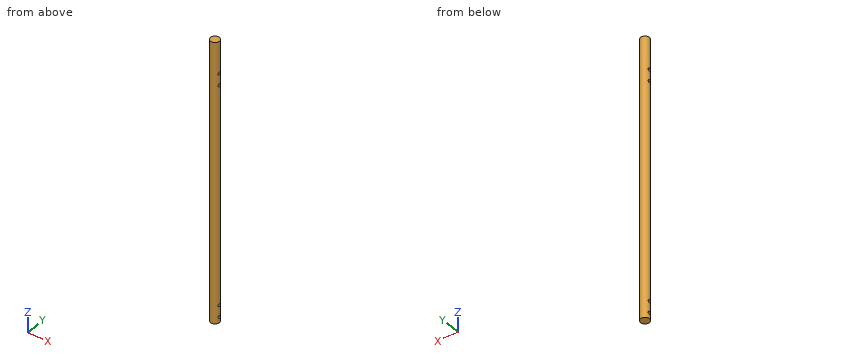
from build123d import *

# Parameters (mm, degrees)
SKETCH1_R                       = 9.525
BOSS_EXTRUDE1_DEPTH             = 609.6
F_1_4_0_25_DIAMETER_HOLE1_D     = 6.35
F_1_4_0_25_DIAMETER_HOLE1_DEPTH = 25.399
F_1_4_0_25_DIAMETER_HOLE1_TIP   = 1.907732465
F_1_4_0_25_DIAMETER_HOLE2_D     = 6.35
F_1_4_0_25_DIAMETER_HOLE2_DEPTH = 25.4
F_1_4_0_25_DIAMETER_HOLE2_TIP   = 1.907732465


with BuildPart() as part:
    # Sketch1 → Boss-Extrude1 (new body)
    with BuildSketch(Plane.XY):
        with Locations(Location((0, 0, 0), (0, 0, 180))):
            Circle(SKETCH1_R)
    extrude(amount=BOSS_EXTRUDE1_DEPTH)

    # 1/4 (0.25) Diameter Hole1
    with Locations(Plane(origin=(-12.7, 0, 514.35), x_dir=(0, 0, -1), z_dir=(-1, 0, 0))):
        with Locations((0, 0), (-25.4, 0)):
            Hole(F_1_4_0_25_DIAMETER_HOLE1_D / 2, depth=F_1_4_0_25_DIAMETER_HOLE1_DEPTH)
            with Locations((0, 0, -(F_1_4_0_25_DIAMETER_HOLE1_DEPTH + F_1_4_0_25_DIAMETER_HOLE1_TIP / 2))):  # 118° drill point
                Cone(0, F_1_4_0_25_DIAMETER_HOLE1_D / 2, F_1_4_0_25_DIAMETER_HOLE1_TIP, mode=Mode.SUBTRACT)

    # 1/4 (0.25) Diameter Hole2
    with Locations(Plane(origin=(-12.7, 0, 38.1), x_dir=(0, 0, -1), z_dir=(-1, 0, 0))):
        with Locations((0, 0), (25.4, 0)):
            Hole(F_1_4_0_25_DIAMETER_HOLE2_D / 2, depth=F_1_4_0_25_DIAMETER_HOLE2_DEPTH)
            with Locations((0, 0, -(F_1_4_0_25_DIAMETER_HOLE2_DEPTH + F_1_4_0_25_DIAMETER_HOLE2_TIP / 2))):  # 118° drill point
                Cone(0, F_1_4_0_25_DIAMETER_HOLE2_D / 2, F_1_4_0_25_DIAMETER_HOLE2_TIP, mode=Mode.SUBTRACT)


solid = part.part
Input: part model. Units: mm. Frame: model coordinates. Round coordinates to 2 decimals unless told otherwise and drop trailing zeros. Write each loop counter-clockwise with the first axis right and the second up, starting at its lowest first coordinate (ties: lowest second). Pieces come first, ordered by that corner, then holes.
1) Contact query for flat-ended pins moving along their axis: P1, Ø8, axis at y = -5, z = 194.5, coming from the -X side; P2, Ø1, axis at y = -4.5, z = 337.5, coming from the -X side; P3, Ø1.5, axis at y = -6.5, z = 63.5, coming from the -X side. Output: stop coordinate, or through.
2) Cut plane B-B (x = 1.75). Return the cut outline in (y, z) (3 decimals), then the cut area to 3 significant figures.
3) Cut plane C-C (z = 149.5). Return the cut outline in (x, y) (3 decimals), then the cut area to 3 significant figures.
4) Cut plane A-A (y = 0). Return the cut outline in (x, z) (3 decimals), then the cut area to 3 significant figures.
5) Ray query, L1, parallel to Y at x = -0.25, z = 514.35 (3 decimals); L2, parallel to Z at x = 2.5, y = 1.5; L3, parallel to X at y = -0.25, z = 519. Return the intervals inside material, ascending.
Geometry says:
1. P1: stops at x = -9.47
1. P2: stops at x = -8.64
1. P3: stops at x = -7.59
2. outline: (-9.363, 0) - (9.363, 0) - (9.363, 609.6) - (-9.363, 609.6) - close; hole circle Ø6.35 at (0, 12.7); hole circle Ø6.35 at (0, 38.1); hole circle Ø6.35 at (0, 514.35); hole circle Ø6.35 at (0, 539.75)
2. area: 11,300 mm2
3. outline: circle Ø19.05 at (0, 0)
3. area: 285 mm2
4. outline: (-9.525, 0) - (9.525, 0) - (9.525, 9.525) - (-9.525, 9.525) - close; (-9.525, 15.875) - (9.525, 15.875) - (9.525, 34.925) - (-9.525, 34.925) - close; (-9.525, 41.275) - (9.525, 41.275) - (9.525, 511.175) - (-9.525, 511.175) - close; (-9.525, 517.525) - (9.525, 517.525) - (9.525, 536.575) - (-9.525, 536.575) - close; (-9.525, 542.925) - (9.525, 542.925) - (9.525, 609.6) - (-9.525, 609.6) - close
4. area: 11,100 mm2
5. L1: y = -9.522 to -3.175, 3.175 to 9.522
5. L2: z = 0 to 9.9, 15.5 to 35.3, 40.9 to 511.55, 517.15 to 536.95, 542.55 to 609.6
5. L3: x = -9.52 to 9.52
